Geometry check sheet. Reference: drawing and pictorial views, mm from the part's lowest x, y, z. A direction names the side the tool comes from. Coordinates: 2 decimals unless noted, no trailing zeros. Write each loop counter-clockwise with the first axis right and the second up, starting at its lowest first coordinate (ties: lowest second). Pieces come first, ordered by that corner, then holes. Notation, with made-up numbers: M 87.25,73.25 L 129.25,73.25 A8 cw 129.25,79.25 Z; hole C -2,-17 d6. An arc over 180 degrees is marked long. One line per item, written item: value.
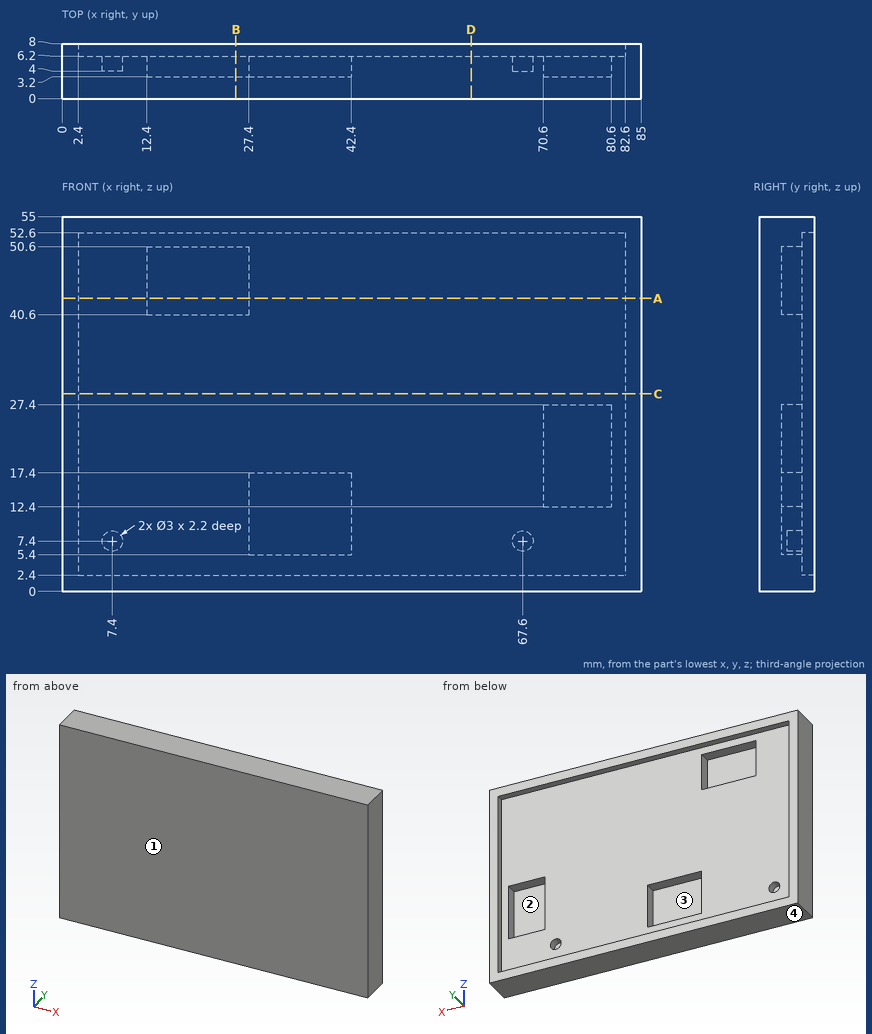
Item 1: Scan lines: line 1 (X direction, y = 5.3, z = 7.4); line 2 (Z direction, x = 71, y = 6); line 3 (X direction, y = 7.75, z = 26). Record each from-to range of solid material in increasing order.
The answers:
line 1: x = 0 to 5.9, 8.9 to 27.4, 42.4 to 66.1, 69.1 to 85
line 2: z = 0 to 12.4, 27.4 to 55
line 3: x = 0 to 2.4, 82.6 to 85
Item 2: Cross-section at A-A, the plane z = 43. Enter the section's corners in (x, y), and give its area (3 significant figures).
The answers:
outline: M 0,0 L 85,0 L 85,8 L 82.6,8 L 82.6,6.2 L 27.4,6.2 L 27.4,3.2 L 12.4,3.2 L 12.4,6.2 L 2.4,6.2 L 2.4,8 L 0,8 Z
area: 491 mm²
Item 3: Go/stop test with flat-tipped pins: P1, Ø3.5, axis at y = 4.5, z = 8.5, coming from the -X side; P2, Ø8, axis at x = 17, z = 46, coming from the +Y side; P3, Ø2.5, axis at x = 67, z = 7, coming from the +Y side. Record where each tip stops, or that it passes through.
The answers:
P1: stops at x = 0
P2: stops at y = 3.2
P3: stops at y = 6.2
Item 4: Access from +Z, -Z, +X, -X, +Y, -Y to the whole of each face (thin tool, end or side, straight path). Record for the marked faces 3 and 4.
The answers:
face 3: +Y
face 4: -Z, +X, -X, +Y, -Y
Item 5: Cross-section at B-B, the plane x = 25.5. Enter the section's corners in (y, z), and give its area (3 significant figures).
The answers:
outline: M 0,0 L 8,0 L 8,2.4 L 6.2,2.4 L 6.2,40.6 L 3.2,40.6 L 3.2,50.6 L 6.2,50.6 L 6.2,52.6 L 8,52.6 L 8,55 L 0,55 Z
area: 320 mm²
Item 6: Cross-section at C-C, the plane z = 29. Enter the section's corners in (x, y), and give its area (3 significant figures).
The answers:
outline: M 0,0 L 85,0 L 85,8 L 82.6,8 L 82.6,6.2 L 2.4,6.2 L 2.4,8 L 0,8 Z
area: 536 mm²
Item 7: Cross-section at D-D, the plane x = 60. Enter the section's corners in (y, z), and give its area (3 significant figures).
The answers:
outline: M 0,0 L 8,0 L 8,2.4 L 6.2,2.4 L 6.2,52.6 L 8,52.6 L 8,55 L 0,55 Z
area: 350 mm²
Item 8: Draft check along X on the marked faces 1 and 2. Enter one of: released by +X, released by -X, zero draft, split by the parting line, or undercut.
The answers:
face 1: zero draft
face 2: undercut
